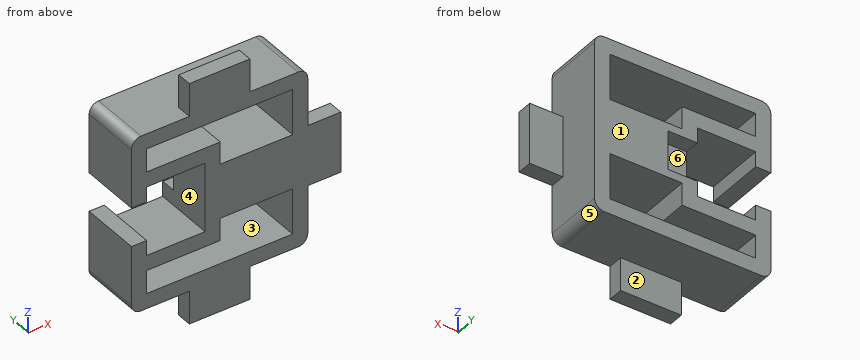
Autodesk Inventor part; units mm, degrees
ref_plane "YZ Plane" through (0, 0, 0) normal (1, 0, 0) x (0, 1, 0)
ref_plane "XZ Plane" through (0, 0, 0) normal (0, 1, 0) x (-1, 0, 0)
ref_plane "XY Plane" through (0, 0, 0) normal (0, 0, 1) x (1, 0, 0)
sketch "Sketch1" plane through (0, 0, 0) normal (0, 1, 0) x (-1, 0, 0)
  line L0 (-9.2329, 9.2329) -> (9.2329, 9.2329)
  line L1 (9.2329, -9.2329) -> (-9.2329, -9.2329)
  line L2 (-9.2329, -9.2329) -> (-9.2329, 9.2329)
  line L3 (-9.2329, 9.2329) -> (9.2329, -9.2329) construction
  line L4 (9.2329, 9.2329) -> (-9.2329, -9.2329) construction
  line L5 (-1.524, 2.032) -> (1.524, 2.032) construction
  line L6 (1.524, 2.032) -> (1.524, -2.032) construction
  line L7 (1.524, -2.032) -> (-1.524, -2.032) construction
  line L8 (-1.524, -2.032) -> (-1.524, 2.032) construction
  line L9 (-1.524, 2.032) -> (1.524, -2.032) construction
  line L10 (1.524, 2.032) -> (-1.524, -2.032) construction
  line L11 (1.524, 2.032) -> (9.2329, 2.032)
  line L12 (9.2329, -2.032) -> (1.524, -2.032)
  line L13 (1.524, -2.032) -> (1.524, 2.032)
  line L14 (9.2329, 9.2329) -> (9.2329, 2.032)
  line L15 (9.2329, -2.032) -> (9.2329, -9.2329)
  point P0 (0, 0)
  dimension "d0" = 18.4658
  dimension "d1" = 3.048
  dimension "d2" = 4.064
extrude "Extrusion1" add sketch "Sketch1" along normal blind 6.35
sketch "Sketch2" plane through (-1.524, 0, -2.032) normal (-1, 0, 0) x (0, 0, 1)
  line L0 (0, 0) -> (4.064, 0)
  line L1 (4.064, 0) -> (4.064, 6.35)
  line L2 (0, 6.35) -> (4.064, 6.35)
  line L3 (0, 0) -> (0, 6.35)
  line L4 (0, 4.7498) -> (4.064, 4.7498)
  line L5 (0, 5.5118) -> (0.762, 6.35)
  line L6 (3.302, 6.35) -> (4.064, 5.5118)
  line L7 (2.032, 4.7498) -> (2.032, 6.35) construction
  point P0 (2.032, 0)
  dimension "d17" = 1.6002
  dimension "d19" = 2.54
  dimension "d21" = 0.762
extrude "Extrusion2" cut sketch "Sketch2" against normal blind 3.048 contours L3 L5 L2 L6 L1 L4
sketch "Sketch6" plane through (0, 6.35, 0) normal (0, 1, 0) x (1, 0, 0)
  line L0 (1.524, -1.27) -> (-1.524, -1.27)
  line L1 (-1.524, -1.27) -> (-1.524, -2.032)
  line L2 (-1.524, -2.032) -> (-9.2329, -2.032)
  line L3 (-9.2329, -2.032) -> (-9.2329, -9.2329)
  line L4 (-9.2329, -9.2329) -> (9.2329, -9.2329)
  line L5 (9.2329, -9.2329) -> (9.2329, 9.2329)
  line L6 (9.2329, 9.2329) -> (-9.2329, 9.2329)
  line L7 (-9.2329, 9.2329) -> (-9.2329, 2.032)
  line L8 (-9.2329, 2.032) -> (-1.524, 2.032)
  line L9 (-1.524, 2.032) -> (-1.524, 1.27)
  line L10 (-1.524, 1.27) -> (1.524, 1.27)
  line L11 (1.524, 1.27) -> (1.524, -1.27)
  line L12 (-7.6454, 7.6454) -> (7.6454, 7.6454)
  line L13 (7.6454, 7.6454) -> (7.6454, -7.6454)
  line L14 (7.6454, -7.6454) -> (-7.6454, -7.6454)
  line L15 (-7.6454, -7.6454) -> (-7.6454, -3.6195)
  line L16 (-7.6454, -3.6195) -> (0.0635, -3.6195)
  line L17 (0.0635, -3.6195) -> (0.0635, -2.8575)
  line L18 (0.0635, -2.8575) -> (3.1115, -2.8575)
  line L19 (3.1115, -2.8575) -> (3.1115, 2.8575)
  line L20 (3.1115, 2.8575) -> (0.0635, 2.8575)
  line L21 (0.0635, 2.8575) -> (0.0635, 3.6195)
  line L22 (0.0635, 3.6195) -> (-7.6454, 3.6195)
  line L23 (-7.6454, 3.6195) -> (-7.6454, 7.6454)
  line L24 (-7.6454, 3.6195) -> (-1.524, 3.6195)
  line L25 (-1.524, 3.6195) -> (-1.524, -3.6195)
  line L26 (-1.524, -3.6195) -> (-7.6454, -3.6195)
  line L27 (-7.6454, -3.6195) -> (-7.6454, 3.6195)
  point P0 (0, 0)
  point P1 (-7.6454, -2.032)
  point P2 (-7.6454, 2.032)
  point P3 (-1.524, 2.032)
  dimension "d22" = 1.5875
extrude "Extrusion5" cut sketch "Sketch6" against normal through all contours L25 L16 L27 L2 | L8 L27 L22 L25
sketch "Sketch7" plane through (0, 6.35, 0) normal (0, 1, 0) x (1, 0, 0)
  line L0 (-7.6454, -3.6195) -> (-7.6454, -2.032)
  line L1 (-7.6454, -2.032) -> (-9.2329, -2.032)
  line L2 (-9.2329, -2.032) -> (-9.2329, -9.2329)
  line L3 (-9.2329, -9.2329) -> (9.2329, -9.2329)
  line L4 (9.2329, -9.2329) -> (9.2329, 9.2329)
  line L5 (9.2329, 9.2329) -> (-9.2329, 9.2329)
  line L6 (-9.2329, 9.2329) -> (-9.2329, 2.032)
  line L7 (-9.2329, 2.032) -> (-7.6454, 2.032)
  line L8 (-7.6454, 2.032) -> (-7.6454, 3.6195)
  line L9 (-7.6454, 3.6195) -> (-1.524, 3.6195)
  line L10 (-1.524, 3.6195) -> (-1.524, 1.27)
  line L11 (-1.524, 1.27) -> (1.524, 1.27)
  line L12 (1.524, 1.27) -> (1.524, -1.27)
  line L13 (1.524, -1.27) -> (-1.524, -1.27)
  line L14 (-1.524, -1.27) -> (-1.524, -3.6195)
  line L15 (-1.524, -3.6195) -> (-7.6454, -3.6195)
  line L16 (-7.6454, 7.6454) -> (7.6454, 7.6454)
  line L17 (7.6454, 7.6454) -> (7.6454, -7.6454)
  line L18 (7.6454, -7.6454) -> (-7.6454, -7.6454)
  line L19 (-7.6454, -7.6454) -> (-7.6454, -5.207)
  line L20 (-7.6454, -5.207) -> (0.0635, -5.207)
  line L21 (0.0635, -5.207) -> (0.0635, -2.8575)
  line L22 (0.0635, -2.8575) -> (3.1115, -2.8575)
  line L23 (3.1115, -2.8575) -> (3.1115, 2.8575)
  line L24 (3.1115, 2.8575) -> (0.0635, 2.8575)
  line L25 (0.0635, 2.8575) -> (0.0635, 5.207)
  line L26 (0.0635, 5.207) -> (-7.6454, 5.207)
  line L27 (-7.6454, 5.207) -> (-7.6454, 7.6454)
  point P0 (0, 0)
  dimension "d25" = 1.5875
extrude "Extrusion6" cut sketch "Sketch7" against normal through all contours L16 L17 L18 L19 L20 L21 L22 L23 L24 L25 L26 L27
sketch "Sketch8" plane through (0, 0, 0) normal (0, -1, 0) x (1, 0, 0)
  line L0 (-3.175, -12.7) -> (3.175, -12.7)
  line L1 (3.175, -12.7) -> (3.175, 12.7)
  line L2 (3.175, 12.7) -> (-3.175, 12.7)
  line L3 (-3.175, 12.7) -> (-3.175, -12.7)
  line L4 (-3.175, -12.7) -> (3.175, 12.7) construction
  line L5 (3.175, -12.7) -> (-3.175, 12.7) construction
  line L6 (0.0635, -5.207) -> (0.0635, -2.8575)
  line L7 (0.0635, -2.8575) -> (3.1115, -2.8575)
  line L8 (3.1115, -2.8575) -> (3.1115, 2.8575)
  line L9 (3.1115, 2.8575) -> (0.0635, 2.8575)
  line L10 (0.0635, 2.8575) -> (0.0635, 5.207)
  line L11 (0.0635, 5.207) -> (-7.6454, 5.207)
  line L12 (-7.6454, 5.207) -> (-7.6454, 7.6454)
  line L13 (-7.6454, 7.6454) -> (7.6454, 7.6454)
  line L14 (7.6454, 7.6454) -> (7.6454, -7.6454)
  line L15 (7.6454, -7.6454) -> (-7.6454, -7.6454)
  line L16 (-7.6454, -7.6454) -> (-7.6454, -5.207)
  line L17 (-7.6454, -5.207) -> (0.0635, -5.207)
  line L18 (-7.6454, 2.032) -> (-7.6454, 3.6195)
  line L19 (-7.6454, 3.6195) -> (-1.524, 3.6195)
  line L20 (-1.524, -3.6195) -> (-1.524, 3.6195)
  line L21 (-1.524, -3.6195) -> (-7.6454, -3.6195)
  line L22 (-7.6454, -3.6195) -> (-7.6454, -2.032)
  line L23 (-9.2329, -2.032) -> (-7.6454, -2.032)
  line L24 (-9.2329, -9.2329) -> (-9.2329, -2.032)
  line L25 (9.2329, -9.2329) -> (-9.2329, -9.2329)
  line L26 (9.2329, 9.2329) -> (9.2329, -9.2329)
  line L27 (-9.2329, 9.2329) -> (9.2329, 9.2329)
  line L28 (-9.2329, 2.032) -> (-9.2329, 9.2329)
  line L29 (-7.6454, 2.032) -> (-9.2329, 2.032)
  line L30 (-12.7, 3.175) -> (-12.7, -3.175)
  line L31 (-12.7, -3.175) -> (12.7, -3.175)
  line L32 (12.7, -3.175) -> (12.7, 3.175)
  line L33 (12.7, 3.175) -> (-12.7, 3.175)
  point P0 (0, 0)
  point P1 (3.175, -9.2329)
  point P2 (-3.175, -9.2329)
  point P3 (9.2329, 3.175)
  point P4 (9.2329, -3.175)
  point P5 (-3.175, 9.2329)
  point P6 (3.175, 9.2329)
  dimension "d28" = 6.35
  dimension "d29" = 25.4
  dimension "d32" = 90
extrude "Extrusion7" add sketch "Sketch8" against normal blind 1.5875 contours L3 L25 L1 L0 | L26 L33 L32 L31 | L27 L3 L2 L1
sketch "Sketch9" plane through (0, 0, 0) normal (0, -1, 0) x (1, 0, 0)
  line L0 (-1.524, -2.032) -> (1.524, -2.032)
  line L1 (0.0635, -5.207) -> (0.0635, -2.8575)
  line L2 (0.0635, -2.8575) -> (3.1115, -2.8575)
  line L3 (3.1115, -2.8575) -> (3.1115, 2.8575)
  line L4 (3.1115, 2.8575) -> (0.0635, 2.8575)
  line L5 (0.0635, 2.8575) -> (0.0635, 5.207)
  line L6 (0.0635, 5.207) -> (-7.6454, 5.207)
  line L7 (-7.6454, 5.207) -> (-7.6454, 7.6454)
  line L8 (-7.6454, 7.6454) -> (7.6454, 7.6454)
  line L9 (7.6454, 7.6454) -> (7.6454, -7.6454)
  line L10 (7.6454, -7.6454) -> (-7.6454, -7.6454)
  line L11 (-7.6454, -7.6454) -> (-7.6454, -5.207)
  line L12 (-7.6454, -5.207) -> (0.0635, -5.207)
  line L13 (-7.6454, 2.032) -> (-7.6454, 3.6195)
  line L14 (-7.6454, 3.6195) -> (-1.524, 3.6195)
  line L15 (-1.524, -3.6195) -> (-1.524, 3.6195)
  line L16 (-1.524, -3.6195) -> (-7.6454, -3.6195)
  line L17 (-7.6454, -3.6195) -> (-7.6454, -2.032)
  line L18 (-9.2329, -2.032) -> (-7.6454, -2.032)
  line L19 (-9.2329, -9.2329) -> (-9.2329, -2.032)
  line L20 (-3.175, -9.2329) -> (-9.2329, -9.2329)
  line L21 (-3.175, -9.2329) -> (-3.175, -12.7)
  line L22 (-3.175, -12.7) -> (3.175, -12.7)
  line L23 (3.175, -12.7) -> (3.175, -9.2329)
  line L24 (9.2329, -9.2329) -> (3.175, -9.2329)
  line L25 (9.2329, -3.175) -> (9.2329, -9.2329)
  line L26 (9.2329, -3.175) -> (12.7, -3.175)
  line L27 (12.7, -3.175) -> (12.7, 3.175)
  line L28 (12.7, 3.175) -> (9.2329, 3.175)
  line L29 (9.2329, 9.2329) -> (9.2329, 3.175)
  line L30 (3.175, 9.2329) -> (9.2329, 9.2329)
  line L31 (3.175, 9.2329) -> (3.175, 12.7)
  line L32 (3.175, 12.7) -> (-3.175, 12.7)
  line L33 (-3.175, 12.7) -> (-3.175, 9.2329)
  line L34 (-9.2329, 9.2329) -> (-3.175, 9.2329)
  line L35 (-9.2329, 2.032) -> (-9.2329, 9.2329)
  line L36 (-7.6454, 2.032) -> (-9.2329, 2.032)
  line L37 (3.1115, -2.8575) -> (7.6454, -2.8575)
  line L38 (7.6454, -2.8575) -> (7.6454, 2.8575)
  line L39 (7.6454, 2.8575) -> (3.1115, 2.8575)
  line L40 (3.1115, 2.8575) -> (3.1115, -2.8575)
  line L41 (3.1115, 2.8575) -> (0.0635, 2.8575)
  point P0 (0, 0)
  point P1 (7.6454, 2.8575)
extrude "Extrusion8" add sketch "Sketch9" against normal up to surface (6.35 mm away) contours L3 L39 L9 L37
sketch "Sketch10" plane through (-1.524, 4.7498, 2.032) normal (-1, 0, 0) x (0, 0, 1)
  line L0 (-0.762, 1.6002) -> (0, 0.762)
  line L1 (0, 0) -> (0, 0.762)
  line L2 (0, 0) -> (-4.064, 0)
  line L3 (-4.064, 0.762) -> (-4.064, 0)
  line L4 (-4.064, 0.762) -> (-3.302, 1.6002)
  line L5 (-5.6515, 1.6002) -> (-3.302, 1.6002)
  line L6 (-5.6515, 1.6002) -> (-5.6515, -4.7498)
  line L7 (-5.6515, -4.7498) -> (1.5875, -4.7498)
  line L8 (1.5875, 1.6002) -> (1.5875, -4.7498)
  line L9 (-0.762, 1.6002) -> (1.5875, 1.6002)
  line L10 (-11.2649, -4.7498) -> (-4.064, -4.7498)
  line L11 (-4.064, -4.7498) -> (-4.064, 1.6002)
  line L12 (-11.2649, 1.6002) -> (-4.064, 1.6002)
  line L13 (-11.2649, -4.7498) -> (-11.2649, 1.6002)
  line L14 (0, -4.7498) -> (7.2009, -4.7498)
  line L15 (7.2009, -4.7498) -> (7.2009, 1.6002)
  line L16 (0, 1.6002) -> (7.2009, 1.6002)
  line L17 (0, -4.7498) -> (0, 1.6002)
  point P0 (-2.032, -4.7498)
extrude "Extrusion9" cut sketch "Sketch10" against normal up to surface (3.048 mm away) contours L9 L17 L0 | L11 L5 L4
fillet "Fillet3" radius 1 4 edges at (-9.2329, 3.175, -9.2329) (-9.2329, 3.175, 9.2329) (9.2329, 3.175, 9.2329) (9.2329, 3.175, -9.2329)
properties part number "hall holder"
The model under review builds one solid part; all positions refer to its coordinate system, in mm. Face numbers are marked on the shaded views. A direction names the side the tool comes from. Round coordinates to 2 decimals unless told otherwise and drop trailing zeros. Order: outer loops, then holes, each group sorted by start corner. A loop starts at its lowest first (then second) coordinate and runs counter-clockwise, first axis right, second up. Notation, with made-up numbers: M 84,27.25 L 120,27.25 A11 cw 120,47.25 Z; hole C 31.5,21.5 d9. An arc over 180 degrees is marked long. Use a Markdown table: item, result.
1) Consider section D-D (x = -5.5). Write out the cut boundary in (y, z), then the cut area to 3 significant figures.
Report:
| item | result |
|---|---|
| outline | M 0,-9.23 L 6.35,-9.23 L 6.35,-7.65 L 0,-7.65 Z; M 0,-5.21 L 6.35,-5.21 L 6.35,-3.62 L 0,-3.62 Z; M 0,3.62 L 6.35,3.62 L 6.35,5.21 L 0,5.21 Z; M 0,7.65 L 6.35,7.65 L 6.35,9.23 L 0,9.23 Z |
| area | 40.3 mm^2 |
2) Wall thickness on line 1 along Z through (x, y) = (2.5, 2.5); line 2 along Z through (x, y) = (-2.5, 1); line 3 along Z through (x, y) = (-6.25, 2.5): over which ranges is each line inside the solid? List them lowest first. Write a range as [from, to].
Report:
| item | result |
|---|---|
| line 1 | [-9.23, -7.65], [-2.86, 2.86], [7.65, 9.23] |
| line 2 | [-12.7, -7.65], [-5.21, -3.62], [3.62, 5.21], [7.65, 12.7] |
| line 3 | [-9.23, -7.65], [-5.21, -3.62], [3.62, 5.21], [7.65, 9.23] |
3) Consider section B-B (y = 5.5). Give the number of separate pieces and of enclosed holes in the cut face, then the cut area to 3 significant figures.
Report:
| item | result |
|---|---|
| separate pieces | 1 |
| enclosed holes | 2 |
| area | 167 mm^2 |
4) Tool access review of the marked faces 1, 2 and 3: name each direction out of +Z, -Z, +X, -X, +Y, -Y from which nothing blocks a thin tool from reaching the whole face with its end or side.
Report:
| item | result |
|---|---|
| face 1 | +Z, -Z, +X, -X, +Y |
| face 2 | -Z, +X, -X, +Y |
| face 3 | +Y, -Y |
5) Insertion check: pin 1 (1 mm diameter, centred on x = -2.5, y = 2.5, fed in from +Z); pin 2 (1.5 mm diameter, centred on x = -0.5, z = 0, fed in from +Y); pin 3 (1.8 mm diameter, centred on x = 0, y = 6, fed in from -Z). Each pin has a flat end and moves straight along its axis. Give the tip position at first contact, or say it passes through.
Report:
| item | result |
|---|---|
| pin 1 | z = 9.23 |
| pin 2 | y = 4.75 |
| pin 3 | z = -9.23 |
6) Draft analysis for pull direction X (two halves, no side actions). For the marked faces 4, 5 and 6, state which applies: released by +X, released by -X, zero draft, split by the parting line, or undercut.
Report:
| item | result |
|---|---|
| face 4 | undercut |
| face 5 | released by +X |
| face 6 | zero draft |
7) Consider section A-A (x = 2.75). Write out the cut boundary in (y, z), then the cut area to 3 significant figures.
Report:
| item | result |
|---|---|
| outline | M 0,-12.7 L 1.59,-12.7 L 1.59,-9.23 L 6.35,-9.23 L 6.35,-7.65 L 0,-7.65 Z; M 0,-2.86 L 6.35,-2.86 L 6.35,2.86 L 0,2.86 Z; M 0,7.65 L 6.35,7.65 L 6.35,9.23 L 1.59,9.23 L 1.59,12.7 L 0,12.7 Z |
| area | 67.5 mm^2 |
8) Consider section C-C (z = 4.5). Write out the cut boundary in (x, y), then the cut area to 3 significant figures.
Report:
| item | result |
|---|---|
| outline | M -9.23,0 L 0.06,0 L 0.06,6.35 L -9.23,6.35 Z; M 7.65,0 L 9.23,0 L 9.23,6.35 L 7.65,6.35 Z |
| area | 69.1 mm^2 |
